Geometry: final body of the model. Coordinates: model frame, mm. A direction names the side the tool comes from. Give positions to 0.01 mm unless a question says otherwise; leave off trailing zeros. Loops run counter-clockwise (first coordinate to the right, second up) from the corner with the lowest first, then second, coordinate; pieces in that order, holes last.
1. Section D-D, the plane z = 14.25. Output: boundary loops of the cut face in (x, y), then the cut area to 3 significant figures.
2. First-contact query: P1, Ø6, axis at y = 3.5, z = 8.5, coming from the -X side; P2, Ø1, axis at y = 3.5, z = 8, coming from the +X side. Flat tips, straight axial feed; report the tip coordinate or a pass-through.
3. Material intervals for line 1 along Z through (x, y) = (-3.5, -1); line 2 along Y through (x, z) = (-2.25, 5); line 3 along Z through (x, y) = (-1, 2), sorted ascending.
4. Section B-B, the plane y = 0. Output: boundary loops of the cut face in (x, z), then the cut area to 3 significant figures.
5. Access query for faces 1 (the face through (0, 5, 7)), 2 (the face through (-0.54, -2.44, 15.74)), 3 (the face through (-0.108, 0.488, -0.986)). Directions: +Z, -Z, +X, -X, +Y, -Y. A direction counts if a zero-diameter tool reaches every point of the face in a straight line with its end or side. Return the directions, or none.
6. Section C-C, the plane x = 0. Output: boundary loops of the cut face in (y, z), then the cut area to 3 significant figures.
7. Section A-A, the plane x = 3. Output: boundary loops of the cut face in (y, z), then the cut area to 3 significant figures.
from build123d import *

# Parameters (mm, degrees)
AUFSATZ_LINEAR_AUSTRAGEN1_DEPTH = 15.2
SKIZZE2_R                       = 2.5
AUFSATZ_LINEAR_AUSTRAGEN2_DEPTH = 1.3
SKIZZE3_R                       = 0.5
AUFSATZ_LINEAR_AUSTRAGEN3_DEPTH = 2
VERRUNDUNG1_R                   = 0.2
SKIZZE4_W                       = 0.3
SKIZZE4_H                       = 4.8
SCHNITT_LINEAR_AUSTRAGEN1_DEPTH = 0.1


with BuildPart() as part:
    # Skizze1 → Aufsatz-Linear austragen1 (new body)
    with BuildSketch(Plane.XY):
        with BuildLine():
            Line((-3.31662479, 5), (3.31662479, 5))
            ThreePointArc((3.31662479, 5), (6, 0), (3.31662479, -5))
            Line((3.31662479, -5), (-3.31662479, -5))
            ThreePointArc((-3.31662479, -5), (-6, 0), (-3.31662479, 5))
        make_face()
    extrude(amount=AUFSATZ_LINEAR_AUSTRAGEN1_DEPTH)

    # Skizze2 → Aufsatz-Linear austragen2 (add)
    with BuildSketch(Plane.XY.offset(15.2)):
        Circle(SKIZZE2_R)
    extrude(amount=AUFSATZ_LINEAR_AUSTRAGEN2_DEPTH)

    # Skizze3 → Aufsatz-Linear austragen3 (add)
    with BuildSketch(Plane(origin=(0, 0, 0), x_dir=(-1, 0, 0), z_dir=(0, 0, -1))):
        with Locations(Location((0, 0, 0), (0, 0, 180))):
            Circle(SKIZZE3_R)
    extrude(amount=AUFSATZ_LINEAR_AUSTRAGEN3_DEPTH)

    # Verrundung1
    verrundung1_edges = [part.edges().sort_by_distance(p)[0] for p in [
        (6, 0, 15.2),
        (0, 5, 15.2),
        (-2.5, 0, 16.5),
        (-6, 0, 15.2),
        (0, 5, 0),
        (6, 0, 0),
        (0, -5, 0),
        (-6, 0, 0),
        (0, -5, 15.2),
    ]]
    fillet(verrundung1_edges, radius=VERRUNDUNG1_R)

    # Skizze4 → Schnitt-Linear austragen1 (cut)
    with BuildSketch(Plane(origin=(0, 5, 0), x_dir=(1, 0, 0), z_dir=(0, 1, 0))):
        with Locations((-2.15, -6.8)):
            Rectangle(SKIZZE4_W, SKIZZE4_H)
        with Locations((2.15, -6.8)):
            Rectangle(SKIZZE4_W, SKIZZE4_H)
    schnitt_linear_austragen1 = extrude(amount=-SCHNITT_LINEAR_AUSTRAGEN1_DEPTH, mode=Mode.SUBTRACT)

    # Spiegeln1: Schnitt-Linear austragen1 across plane
    add(schnitt_linear_austragen1.mirror(Plane.ZX), mode=Mode.SUBTRACT)


solid = part.part
Answers below:
1. outline: (-3.32, -5) - (3.32, -5) arc R6 ccw to (3.32, 5) - (-3.32, 5) arc R6 ccw to start
1. area: 104 mm2
2. P1: stops at x = -5.98
2. P2: stops at x = 5.2
3. line 1: z = 0 to 15.2
3. line 2: y = -4.9 to 4.9
3. line 3: z = 0 to 16.5
4. outline: (-6, 0.2) arc R0.2 ccw to (-5.8, 0) - (-0.5, 0) - (-0.5, -2) - (0.5, -2) - (0.5, 0) - (5.8, 0) arc R0.2 ccw to (6, 0.2) - (6, 15) arc R0.2 ccw to (5.8, 15.2) - (2.5, 15.2) - (2.5, 16.3) arc R0.2 ccw to (2.3, 16.5) - (-2.3, 16.5) arc R0.2 ccw to (-2.5, 16.3) - (-2.5, 15.2) - (-5.8, 15.2) arc R0.2 ccw to (-6, 15) - close
4. area: 191 mm2
5. face 1: +Z, -Z, +X, -X, +Y
5. face 2: +Z
5. face 3: -Z
6. outline: (-5, 0.2) arc R0.2 ccw to (-4.8, 0) - (-0.5, 0) - (-0.5, -2) - (0.5, -2) - (0.5, 0) - (4.8, 0) arc R0.2 ccw to (5, 0.2) - (5, 15) arc R0.2 ccw to (4.8, 15.2) - (2.5, 15.2) - (2.5, 16.3) arc R0.2 ccw to (2.3, 16.5) - (-2.3, 16.5) arc R0.2 ccw to (-2.5, 16.3) - (-2.5, 15.2) - (-4.8, 15.2) arc R0.2 ccw to (-5, 15) - close
6. area: 160 mm2
7. outline: (-5, 0.2) arc R0.2 ccw to (-4.8, 0) - (4.8, 0) arc R0.2 ccw to (5, 0.2) - (5, 15) arc R0.2 ccw to (4.8, 15.2) - (-4.8, 15.2) arc R0.2 ccw to (-5, 15) - close
7. area: 152 mm2
